The figure shows three views and two pictorial views of one solid part (mm, origin at its lowest corner). Answer the questions. Round coordinates to 2 decimals unless told otherwise and drop trailing zeros. Order: outer loops, then holes, each group sorted by start corner. A loop starts at its lowest first (then second) coordinate and runs counter-clockwise, first axis right, second up. Notation, with made-up numbers: M 4.25,35.25 L 60.25,35.25 A20 ccw 60.25,40.25 Z; hole C -26.5,5.25 d9. An arc over 180 degrees is marked long. Return JSON: item names as keys, results as strings.
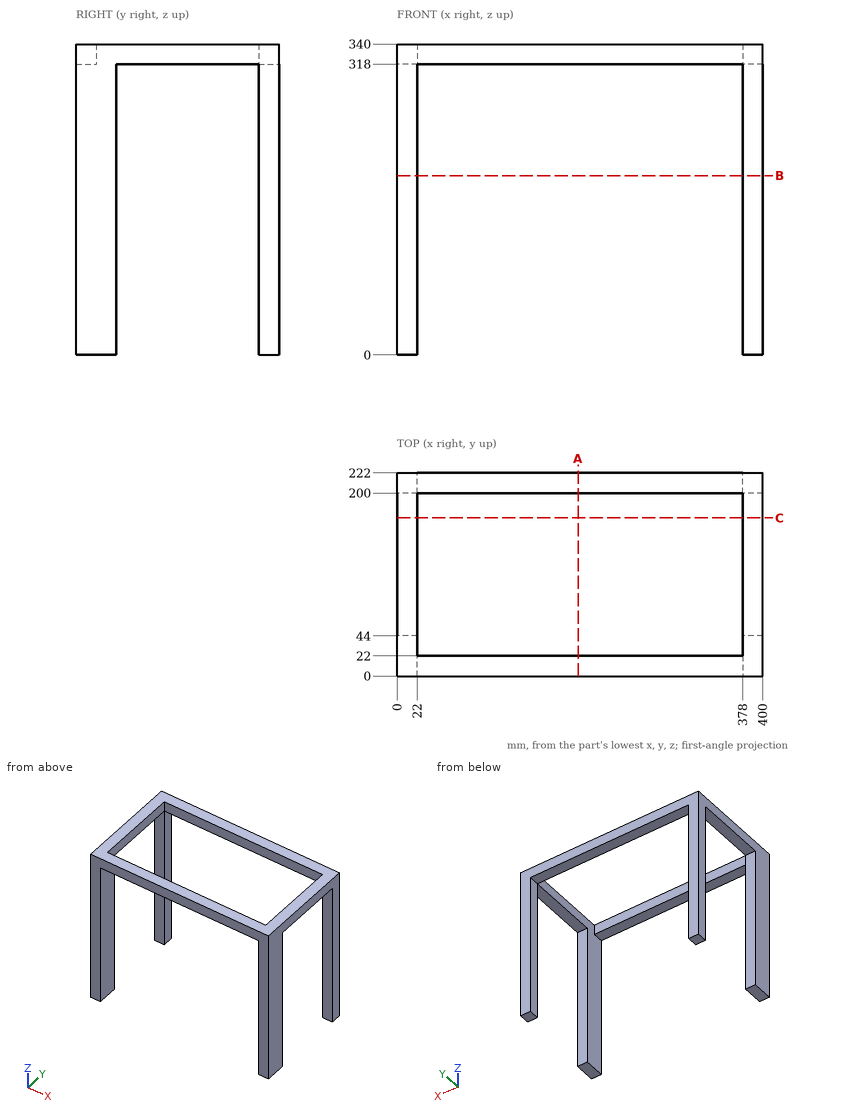
Item 1: This flat-tipped pin is pushed along its axis until it touches: pin 1 (11 mm diameter, centred on x = 221, y = 10, fed in from -Z). Where does it stop, or does it pass through?
Output:
{"pin 1": "stops at z = 318"}
Item 2: Find section C-C (y = 173). Determine the outline of the cut face in (x, z).
Output:
{"outline": "M 0,318 L 22,318 L 22,340 L 0,340 Z; M 378,318 L 400,318 L 400,340 L 378,340 Z"}
Item 3: Find section B-B (z = 196). Determine the outline of the cut face in (x, y), plus the area to 3 significant figures.
Output:
{"outline": "M 0,0 L 22,0 L 22,44 L 0,44 Z; M 0,200 L 22,200 L 22,222 L 0,222 Z; M 378,0 L 400,0 L 400,44 L 378,44 Z; M 378,200 L 400,200 L 400,222 L 378,222 Z", "area": "2,900 mm^2"}
Item 4: Find section A-A (x = 198). Determine the outline of the cut face in (y, z).
Output:
{"outline": "M 0,318 L 22,318 L 22,340 L 0,340 Z; M 200,318 L 222,318 L 222,340 L 200,340 Z"}
Item 5: Consider line 1 along X through (y, z) = (204.5, 281); line 2 along Z through (x, y) = (339.5, 12). Determine where each line is inside the solid, lowest interval first. Write a range as [from, to].
Output:
{"line 1": "x = [0, 22], [378, 400]", "line 2": "z = [318, 340]"}
